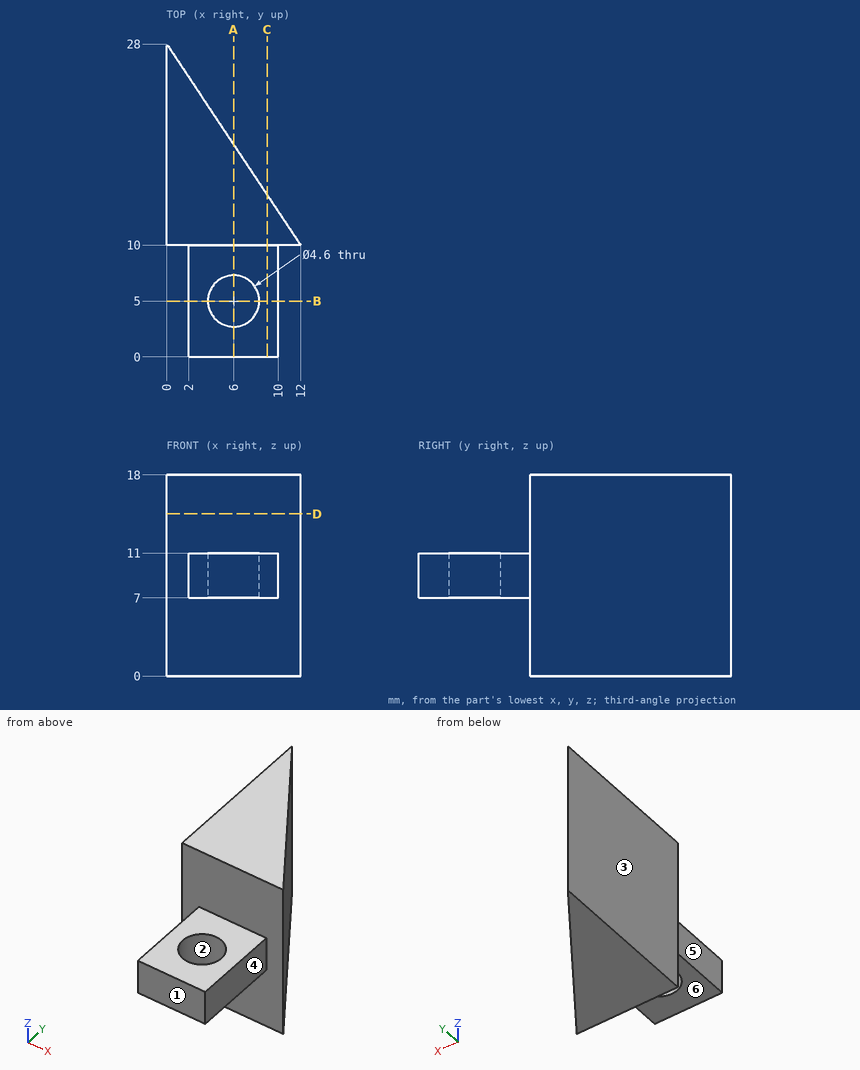
The figure shows three views and two pictorial views of one solid part (mm, origin at its lowest corner). Answer the questions. A direction names the side the tool comes from. Give positions to 0.01 mm unless a question says otherwise; leave off trailing zeros. Loops run counter-clockwise (first coordinate to the right, second up) from the corner with the lowest first, then second, coordinate; pieces in that order, holes last. Notation, with made-up numbers: (87.5, 54) - (116.5, 54) arc R25 ccw to (116.5, 67) - close; hole circle Ø7 at (64, 1.5). An arc over 180 degrees is marked (long way). Use one line per item in the form item = value.
1. Section C-C on x = 9 is taken. Give the vertices of the cut face in (y, z).
Calculated:
outline = (0, 7) - (10, 7) - (10, 0) - (14.5, 0) - (14.5, 18) - (10, 18) - (10, 11) - (0, 11) - close
2. Section A-A on x = 6 is taken. Give the vertices of the cut face in (y, z).
Calculated:
outline = (0, 7) - (2.7, 7) - (2.7, 11) - (0, 11) - close; (7.3, 7) - (10, 7) - (10, 0) - (19, 0) - (19, 18) - (10, 18) - (10, 11) - (7.3, 11) - close
3. Section B-B on y = 5 is taken. Give the vertices of the cut face in (x, z).
Calculated:
outline = (2, 7) - (3.7, 7) - (3.7, 11) - (2, 11) - close; (8.3, 7) - (10, 7) - (10, 11) - (8.3, 11) - close
4. Section D-D on z = 14.5 is taken. Give the vertices of the cut face in (x, y).
Calculated:
outline = (0, 10) - (12, 10) - (0, 28) - close
5. Which of the six approach directions +Z, -Z, +X, -X, +Y, -Y give full straight-line access (tool end or side, diameter ignored) to the marked faces 4, 5 and 6?
Calculated:
face_4 = +Z, -Z, +X, -Y
face_5 = +Z, -Z, -X, -Y
face_6 = -Z, +X, -X, -Y
6. Given pin 1 Ø3 at (y, z) = (14, 16) entering from +X; pin 2 Ø2 at (y, z) = (5, 8.5) entering from -X; pin 3 Ø1.2 at (y, z) = (6.5, 8.5) entering from +X, each flat-ended and moving along its own axis, determine where each tip first touches the part or whether it passes through.
Calculated:
pin_1 = 10.33
pin_2 = 2
pin_3 = 10
7. Find the intervals of material crossed by line 1 along Y through (x, z) = (6, 8.4); line 2 along Y through (x, z) = (4.75, 2.75) (3 decimals); line 3 along X through (y, z) = (14.5, 6.5), in increasing order. Write a range as [from, to].
Calculated:
line_1 = [0, 2.7], [7.3, 19]
line_2 = [10, 20.875]
line_3 = [0, 9]
8. The mould has two halves that part along Y. Classify the marked faces 1, 2 and 3: pulls with the +Y half, pulls with the -Y half, needs draft (parallel to the pull), parting line crosses it, or undercut.
Calculated:
face_1 = pulls with the -Y half
face_2 = undercut
face_3 = needs draft
